Print and shaded views of the part. All mm, measured from the part's lowest x, y and z. Coordinates: 2 decimals unless noted, no trailing zeros. Loops run counter-clockwise (first coordinate to the right, second up) from the corner with the lowest first, then second, coordinate; pieces in that order, holes last. Notation, with made-up numbers: (-28, -32.75) -> (-24, -32.75) arc R16 cw to (-24, -21.75) -> close; hole circle Ø7 at (58.5, -37.75). An arc over 180 degrees is marked (long way). One line per question, with ' | ' between items. Start each with the question number.
1) Probe L1, parallel to Y at x = 34.5, z = 7.25; L2, parallel to X at y = 9.25, z = 9.25; L3, parallel to Z at x = 49.5, y = 9.5. List the from-to ranges inside material, lowest first. Write a range as from..to.
2) Cut at B-B (z = 8.5). List the corners of the cut face in (x, y).
3) Drop flat-ended pins along their axis: pin 1 (1 mm diameter, centred on x = 29.5, z = 5, fed in from -Y); pin 2 (1.5 mm diameter, centred on x = 49.5, y = 7, fed in from +Z); pin 3 (5 mm diameter, centred on y = 3, z = 11.5, fed in from -X). Give the stop position or say it passes through.
4) Cut at A-A (x = 51). List the corners of the cut face in (y, z) (1 decimal).
5) Two-plate mould, pull along X, no slides. Class the marked faces 1 and 2: released by +X, released by -X, zero draft, split by the parting line, or undercut.
6) Cut at C-C (y = 18.5). List the corners of the cut face in (x, z).
7) Cut at D-D (x = 10). List the corners of the cut face in (y, z) (1 decimal).
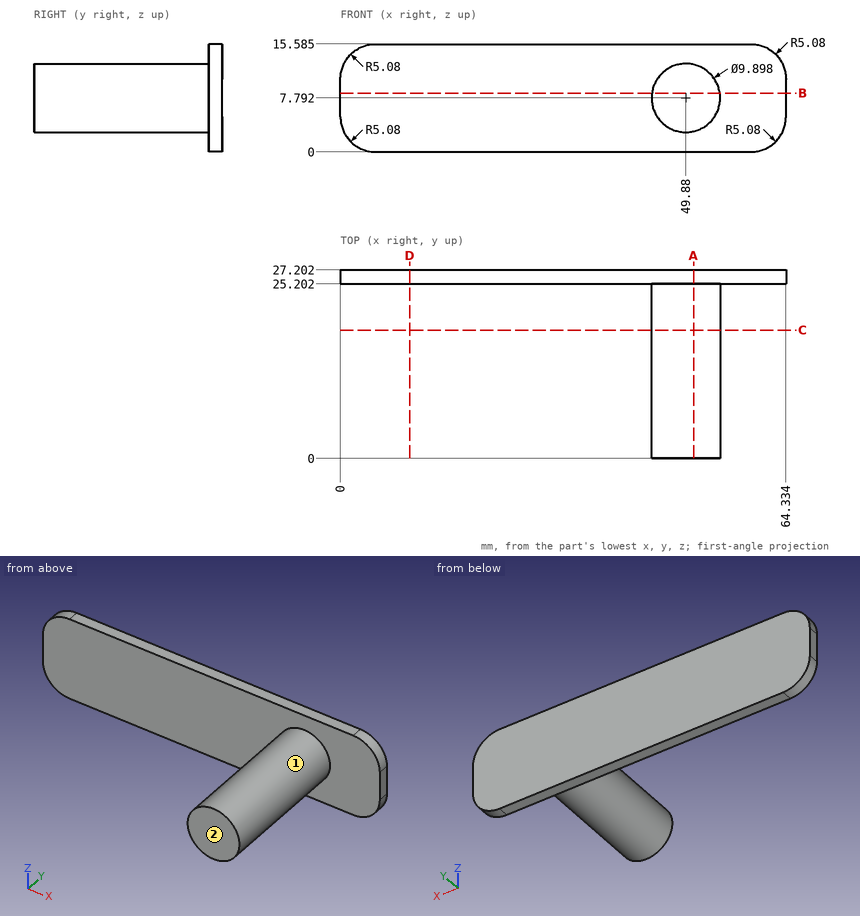
Reported:
1) L1: y = 25.2..27.2 | L2: x = 45.15..54.61 | L3: z = 2.86..12.73
2) outline: (0, 25.2) -> (44.98, 25.2) -> (44.98, 0) -> (54.78, 0) -> (54.78, 25.2) -> (64.33, 25.2) -> (64.33, 27.2) -> (0, 27.2) -> close
3) pin 1: stops at y = 25.2 | pin 2: stops at z = 12.74 | pin 3: stops at x = 45.08
4) outline: (0, 3) -> (25.2, 3) -> (25.2, 0) -> (27.2, 0) -> (27.2, 15.6) -> (25.2, 15.6) -> (25.2, 12.6) -> (0, 12.6) -> close
5) face 1: split by the parting line | face 2: zero draft
6) outline: circle Ø9.9 at (49.88, 7.79)
7) outline: (25.2, 0) -> (27.2, 0) -> (27.2, 15.6) -> (25.2, 15.6) -> close
